The figure shows three views and two pictorial views of one solid part (mm, origin at its lowest corner). Answer the questions. Coordinates: 2 decimals unless noted, no trailing zeros. Loops run counter-clockwise (first coordinate to the right, second up) from the corner with the lowest first, then second, coordinate; pieces in that order, holes last. Notation, with made-up numbers: M 23,1.25 L 37,1.25 A30 cw 37,29.25 Z; hole C -31.5,60.25 d1. An arc over 180 degrees is marked long. One line per item, written item: value. Start each with the question number.
1. Flat-ended cylindrical pins translate along their axes: pin 1 (1 mm diameter, centred on y = 18.5, z = 53.5, fed in from +X) (1 decimal); pin 2 (6 mm diameter, centred on y = 6, z = 22.5, fed in from +X); pin 3 (1.9 mm diameter, centred on x = 45, y = 12.7, fed in from +Z). Find the tip coordinate at first contact, or state that the pin passes through.
2. The part is cut by section B-B (x = 45). Write down the section's boundary in (y, z) (1 decimal).
3. Consider probe 1 along Y at (x, z) = (45, 59); probe 2 along Z at (x, y) = (45, 24.5) (1 decimal); probe 3 along X at (y, z) = (8.75, 32). Determine where each line is inside the solid, lowest interval first.
4. The part is cut by section C-C (y = 12.7). Write down the section's boundary in (x, z) (1 decimal).
5. The part is cut by section A-A (z = 42). Write down the section's boundary in (x, y) (1 decimal).
6. Determine the mould class of the marked faces 1, 2 and 3 for opening direction X: +X half, -X half, draft (parallel to the pull), parting line (faces both ways), or undercut.
7. The part is cut by section D-D (z = 54). Write down the section's boundary in (x, y) (1 decimal).
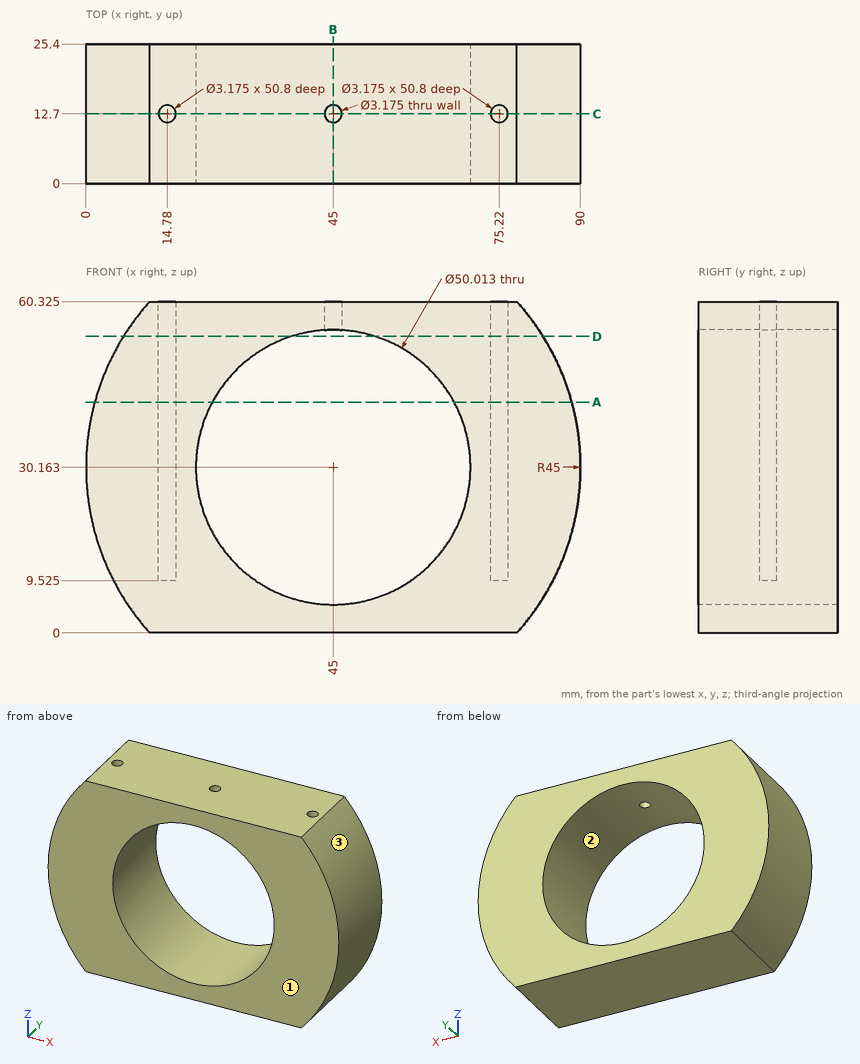
Answer block:
1. pin 1: stops at x = 83.8
1. pin 2: stops at x = 89.76
1. pin 3: stops at z = 5.17
2. outline: M 0,0 L 25.4,0 L 25.4,5.2 L 0,5.2 Z; M 0,55.2 L 11.1,55.2 L 11.1,60.3 L 0,60.3 Z; M 14.3,55.2 L 25.4,55.2 L 25.4,60.3 L 14.3,60.3 Z
3. probe 1: y = 0 to 11.11, 14.29 to 25.4
3. probe 2: z = 0 to 5.2, 55.2 to 60.3
3. probe 3: x = 0.04 to 20.06, 69.94 to 89.96
4. outline: M 11.6,0 L 78.4,0 A45 ccw 78.4,60.3 L 76.8,60.3 L 76.8,9.5 L 73.6,9.5 L 73.6,60.3 L 46.6,60.3 L 46.6,55.1 A25 cw long 43.4,55.1 L 43.4,60.3 L 16.4,60.3 L 16.4,9.5 L 13.2,9.5 L 13.2,60.3 L 11.6,60.3 A45 ccw Z
5. outline: M 1.6,0 L 23,0 L 23,25.4 L 1.6,25.4 Z; M 67,0 L 88.4,0 L 88.4,25.4 L 67,25.4 Z; hole C 14.8,12.7 d3.2; hole C 75.2,12.7 d3.2
6. face 1: draft
6. face 2: undercut
6. face 3: +X half
7. outline: M 6.8,0 L 37.4,0 L 37.4,25.4 L 6.8,25.4 Z; M 52.6,0 L 83.2,0 L 83.2,25.4 L 52.6,25.4 Z; hole C 14.8,12.7 d3.2; hole C 75.2,12.7 d3.2
